Geometry check sheet. Reference: the model listing, model coordinates, mm. A direction names the side the tool comes from. Coordinates: 2 decimals unless noted, no trailing zeros. Order: outer loops, then holes, each group sorted by start corner. A loop starts at its lowest first (then second) coordinate and runs counter-clockwise, first axis right, second up. Notation, with made-up numbers: (13.25, -16.75) - (47.25, -16.75) arc R19 ccw to (47.25, -4.75) - close; hole circle Ø10 at (-12, 27.5). An arc over 180 degrees is marked (long way). Put each result on its own line as item: value.
from build123d import *

# Parameters (mm, degrees)
SKETCH_1_W      = 58
SKETCH_1_H      = 46
SKETCH_1_R      = 17.5
SKETCH_1_R_2    = 2
EXTRUDE_1_DEPTH = 6
SKETCH_2_W      = 12
SKETCH_2_H      = 30
SKETCH_2_R      = 2
EXTRUDE_2_DEPTH = 6
CHAMFER_1_SIZE  = 2


with BuildPart() as part:
    # 草图1 → 凸台-拉伸1 (new body)
    with BuildSketch(Plane(origin=(0, 0, 0), x_dir=(1, 0, 0), z_dir=(0, 1, 0))):
        Rectangle(SKETCH_1_W, SKETCH_1_H)
        with Locations(Location((0, 0, 0), (0, 0, 270))):
            Circle(SKETCH_1_R, mode=Mode.SUBTRACT)
        with Locations(Location((-17.67766953, 17.67766953, 0), (0, 0, 270))):
            Circle(SKETCH_1_R_2, mode=Mode.SUBTRACT)
        with Locations(Location((-17.67766953, -17.67766953, 0), (0, 0, 270))):
            Circle(SKETCH_1_R_2, mode=Mode.SUBTRACT)
        with Locations(Location((17.67766953, 17.67766953, 0), (0, 0, 270))):
            Circle(SKETCH_1_R_2, mode=Mode.SUBTRACT)
        with Locations(Location((17.67766953, -17.67766953, 0), (0, 0, 270))):
            Circle(SKETCH_1_R_2, mode=Mode.SUBTRACT)
        with Locations(Location((-25, 5.5, 0), (0, 0, 270))):
            Circle(SKETCH_1_R_2, mode=Mode.SUBTRACT)
        with Locations(Location((-25, -9, 0), (0, 0, 270))):
            Circle(SKETCH_1_R_2, mode=Mode.SUBTRACT)
        with Locations(Location((25, -9, 0), (0, 0, 270))):
            Circle(SKETCH_1_R_2, mode=Mode.SUBTRACT)
        with Locations(Location((25, 5.5, 0), (0, 0, 270))):
            Circle(SKETCH_1_R_2, mode=Mode.SUBTRACT)
    extrude(amount=EXTRUDE_1_DEPTH)

    # 草图2 → 凸台-拉伸2 (add)
    # profile 1 of 2: a face of its own
    with BuildSketch(Plane(origin=(0, 0, 0), x_dir=(1, 0, 0), z_dir=(0, 1, 0))):
        with Locations((-23, 38)):
            Rectangle(SKETCH_2_W, SKETCH_2_H)
        with Locations(Location((-23, 38, 0), (0, 0, 270))):
            Circle(SKETCH_2_R, mode=Mode.SUBTRACT)
    # profile 2 of 2: a face of its own
    with BuildSketch(Plane(origin=(0, 0, 0), x_dir=(1, 0, 0), z_dir=(0, 1, 0))):
        with Locations((23, 38)):
            Rectangle(SKETCH_2_W, SKETCH_2_H)
        with Locations(Location((23, 38, 0), (0, 0, 90))):
            Circle(SKETCH_2_R, mode=Mode.SUBTRACT)
    extrude(amount=EXTRUDE_2_DEPTH)

    # 倒角1
    chamfer_1_edges = [part.edges().sort_by_distance(p)[0] for p in [
        (25, 6, 7),
        (-25, 6, 7),
        (-25, 6, -7.5),
        (17.67766953, 6, -19.67766953),
        (-17.67766953, 6, 15.67766953),
        (-17.67766953, 6, -19.67766953),
        (17.67766953, 6, 15.67766953),
        (25, 6, -7.5),
    ]]
    chamfer(chamfer_1_edges, length=CHAMFER_1_SIZE - 0.0001)  # a hair under: the kernel refuses the full size


solid = part.part
Q1. Section check C-C on z = -5.5. State how many separate pieces and enclosed holes the cut face has, then the cut area to 3 significant figures.
Answer block:
separate pieces: 4
enclosed holes: 0
area: 92.6 mm^2
Q2. Access from +Z, -Z, +X, -X, +Y, -Y to the whole of each face (thin tool, end or side, straight path). Record for faces 1 (the flat face through (0, 3, -23)), 2 (the flat face through (12, 6, -16)).
Answer block:
face 1: -Z, +Y, -Y
face 2: +Z, -Z, +X, -X, +Y
Q3. Depth check by flat-ended pin: pin 1 Ø6.5 at (x, z) = (17.68, -17.68) entering from +Y; pin 2 Ø2 at (x, y) = (-7, 3) entering from -Z; pin 3 Ø4.5 at (x, z) = (17.68, 17.68) entering from +Y. Enter the tip coordinate at first touch or a pass-through.
Answer block:
pin 1: stops at y = 5.25
pin 2: stops at z = -23
pin 3: stops at y = 4.25
Q4. Section check B-B on x = 0. Record the boundary of the cut face in (y, z), then the cut area to 3 significant figures.
Answer block:
outline: (0, -23) - (6, -23) - (6, -17.5) - (0, -17.5) - close; (0, 17.5) - (6, 17.5) - (6, 23) - (0, 23) - close
area: 66.0 mm^2
Q5. Section check A-A on z = -34.5. Record the boundary of the cut face in (x, y), then the cut area to 3 significant figures.
Answer block:
outline: (-29, 0) - (-17, 0) - (-17, 6) - (-29, 6) - close; (17, 0) - (29, 0) - (29, 6) - (17, 6) - close
area: 144 mm^2
Q6. Draft check along Z on faces 3 (the flat face through (-17, 3, -38)), 4 (the flat face through (23, 3, -53)), 5 (the cylindrical face through (23, 3, -36)), 6 (the cylindrical face through (-23, 3, -40)). Enter one of: pulls with the +Z half, pulls with the -Z half, needs draft (parallel to the pull), parting line crosses it, or undercut.
Answer block:
face 3: needs draft
face 4: pulls with the -Z half
face 5: undercut
face 6: undercut
Q7. Thickness scan on L1, parallel to X at y = 3.3, z = -38; L2, parallel to Z at x = -26, y = 4.1; L3, parallel to X at y = 3, z = -19.5. Record the ranges inside material, lowest first. Write a range as [from, to].
Answer block:
L1: x = [-29, -25], [-21, -17], [17, 21], [25, 29]
L2: z = [-53, -7.35], [-3.65, 7.15], [10.85, 23]
L3: x = [-29, -18.5], [-16.85, 16.85], [18.5, 29]
